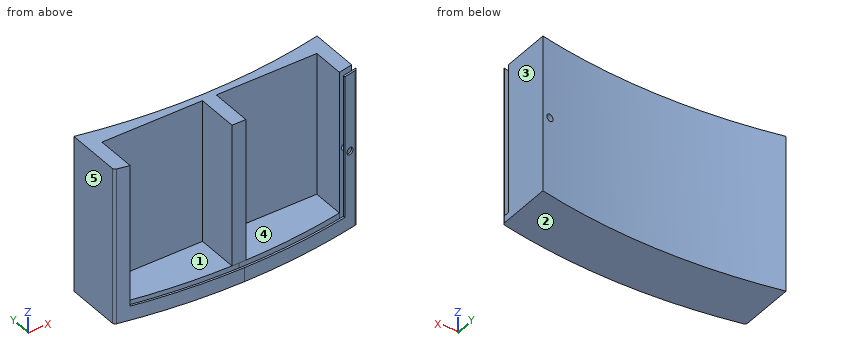
```python
from build123d import *

# Parameters (mm, degrees)
BOSS_EXTRUDE2_DEPTH     = 279.4
CUT_EXTRUDE1_DEPTH      = 279.4
FILLET1_R               = 2.54
SKETCH7_W               = 192.0875
SKETCH7_H               = 254
CUT_EXTRUDE2_DEPTH      = 44.45
SKETCH8_W               = 6.173248721
SKETCH8_H               = 35.639061591
BOSS_EXTRUDE3_DEPTH     = 258.064
CUT_EXTRUDE3_DEPTH      = 260.35
CUT_EXTRUDE3_DEPTH_BACK = 6.35
CUT_EXTRUDE4_DEPTH      = 260.35
CUT_EXTRUDE4_DEPTH_BACK = 6.35
BOSS_EXTRUDE4_DEPTH     = 254
SKETCH18_R              = 3.175
CUT_EXTRUDE5_DEPTH      = 71.12


with BuildPart() as part:
    # CrossSection → Boss-Extrude2 (new body)
    with BuildSketch(Plane.XY):
        with BuildLine():
            Line((108.74375, 11.322324676), (108.74375, -50.8))
            Line((108.74375, -50.8), (-108.74375, -50.8))
            Line((-108.74375, -50.8), (-108.74375, 11.322324676))
            ThreePointArc((-108.74375, 11.322324676), (0, 0), (108.74375, 11.322324676))
        make_face()
    extrude(amount=BOSS_EXTRUDE2_DEPTH)

    # Sketch4 → Cut-Extrude1 (cut)
    with BuildSketch(Plane(origin=(0, 0, 0), x_dir=(-1, 0, 0), z_dir=(0, 0, -1))):
        with BuildLine():
            ThreePointArc((0, -50.8), (-54.665798723, -47.96178867), (-108.74375, -39.477675324))
            Line((-108.74375, -39.477675324), (-108.74375, -50.8))
            Line((-108.74375, -50.8), (0, -50.8))
        make_face()
        with BuildLine():
            ThreePointArc((108.74375, -39.477675324), (54.665798723, -47.96178867), (0, -50.8))
            Line((0, -50.8), (108.74375, -50.8))
            Line((108.74375, -50.8), (108.74375, -39.477675324))
        make_face()
    extrude(amount=-CUT_EXTRUDE1_DEPTH, mode=Mode.SUBTRACT)

    # Fillet1
    fillet1_edges = [part.edges().sort_by_distance(p)[0] for p in [
        (108.74375, -39.477675324, 139.7),
        (-108.74375, -39.477675324, 139.7),
    ]]
    fillet(fillet1_edges, radius=FILLET1_R)

    # Sketch7 → Cut-Extrude2 (cut)
    with BuildSketch(Plane(origin=(0, -50.8, 0), x_dir=(1, 0, 0), z_dir=(0, 1, 0))):
        with Locations((0, -139.7)):
            Rectangle(SKETCH7_W, SKETCH7_H)
    extrude(amount=CUT_EXTRUDE2_DEPTH, mode=Mode.SUBTRACT)

    # Sketch8 → Boss-Extrude3 (add)
    with BuildSketch(Plane.XY.offset(12.7)):
        with Locations((3.086624361, -24.169530796)):
            Rectangle(SKETCH8_W, SKETCH8_H)
        with Locations((-3.086624361, -24.169530796)):
            Rectangle(SKETCH8_W, SKETCH8_H)
    extrude(amount=BOSS_EXTRUDE3_DEPTH)

    # Sketch13 → Cut-Extrude3 (cut, two sides: drawn at the far end of the back side and taken through both)
    with BuildSketch(Plane.XY.offset(12.7).offset(-CUT_EXTRUDE3_DEPTH_BACK)):
        with BuildLine():
            ThreePointArc((-96.04375, -40.123592373), (-48.223527841, -46.727181022), (0, -48.934530782))
            Line((0, -48.934530782), (0, -43.854530782))
            ThreePointArc((0, -43.854530782), (-48.223527841, -41.647181022), (-96.04375, -35.043592373))
            Line((-96.04375, -35.043592373), (-96.04375, -37.583592373))
            Line((-96.04375, -37.583592373), (-96.04375, -40.123592373))
        make_face()
        with BuildLine():
            Line((0, -43.854530782), (0, -48.934530782))
            ThreePointArc((0, -48.934530782), (48.223527841, -46.727181022), (96.04375, -40.123592373))
            Line((96.04375, -40.123592373), (96.04375, -37.583592373))
            Line((96.04375, -37.583592373), (96.04375, -35.043592373))
            ThreePointArc((96.04375, -35.043592373), (48.223527841, -41.647181022), (0, -43.854530782))
        make_face()
    extrude(amount=CUT_EXTRUDE3_DEPTH + CUT_EXTRUDE3_DEPTH_BACK, mode=Mode.SUBTRACT)

    # Sketch14 → Cut-Extrude4 (cut, two sides: drawn at the far end of the back side and taken through both)
    with BuildSketch(Plane(origin=(0, 0, 266.7), x_dir=(-1, 0, 0), z_dir=(0, 0, -1)).offset(-CUT_EXTRUDE4_DEPTH_BACK)):
        with BuildLine():
            Line((96.04375, -35.043592373), (96.04375, -40.123592373))
            ThreePointArc((96.04375, -40.123592373), (-28.026510339, -48.189989717), (-150.541934286, -27.012946445))
            Line((-150.541934286, -27.012946445), (-150.541934286, -21.932946445))
            ThreePointArc((-150.541934286, -21.932946445), (-28.026510339, -43.109989717), (96.04375, -35.043592373))
        make_face()
    extrude(amount=CUT_EXTRUDE4_DEPTH + CUT_EXTRUDE4_DEPTH_BACK, mode=Mode.SUBTRACT)

    # Sketch15 → Boss-Extrude4 (add)
    with BuildSketch(Plane(origin=(0, 0, 266.7), x_dir=(-1, 0, 0), z_dir=(0, 0, -1))):
        with BuildLine():
            Line((6.173248721, -43.818432493), (6.173248721, -41.989061591))
            Line((6.173248721, -41.989061591), (-6.173248721, -41.989061591))
            Line((-6.173248721, -41.989061591), (-6.173248721, -43.818432493))
            ThreePointArc((-6.173248721, -43.818432493), (0, -43.854530782), (6.173248721, -43.818432493))
        make_face()
    extrude(amount=BOSS_EXTRUDE4_DEPTH)

    # Sketch18 → Cut-Extrude5 (cut)
    with BuildSketch(Plane(origin=(0, -50.8, 0), x_dir=(1, 0, 0), z_dir=(0, 1, 0))):
        with Locations(Location((101.380501252, -209.55, 0), (0, 0, 90))):
            Circle(SKETCH18_R)
        with Locations(Location((101.380501252, -69.85, 0), (0, 0, 90))):
            Circle(SKETCH18_R)
    extrude(amount=CUT_EXTRUDE5_DEPTH, mode=Mode.SUBTRACT)


with BuildPart() as body_2:
    # Split2: the piece on the far side of the plane
    add(part.part)
    split(bisect_by=Plane.XY.offset(139.7), keep=Keep.BOTTOM)


with BuildPart() as part_1:
    add(part.part)

    # Split2
    split(bisect_by=Plane.XY.offset(139.7), keep=Keep.TOP)


solid = body_2.part
```
Verification items for the finished model (mm, model axes). Face numbers are marked on the shaded views. A direction names the side the tool comes from. Give positions to 0.01 mm unless a question says otherwise; leave off trailing zeros. Order: outer loops, then holes, each group sorted by start corner. A loop starts at its lowest first (then second) coordinate and runs counter-clockwise, first axis right, second up. Notation, with made-up numbers: (59.25, 3) -> (110.25, 3) arc R32 cw to (110.25, 41) -> close; hole circle Ø2 at (38.25, 25). An arc over 180 degrees is marked (long way). Use a Markdown table: item, result.
1) Depth check by flat-ended pin: pin 1 Ø6 at (x, y) = (48.5, -25.5) entering from +Z; pin 2 Ø1.5 at (x, y) = (64.5, -25.5) entering from -Z; pin 3 Ø4 at (x, z) = (-34.5, 29.5) entering from -Y; pin 4 Ø3 at (x, z) = (-83.5, 86.5) entering from +Y. Enter the tip coordinate at first touch or a pass-through.
Results:
| item | result |
|---|---|
| pin 1 | z = 12.7 |
| pin 2 | z = 0 |
| pin 3 | y = -6.35 |
| pin 4 | y = 6.89 |
2) Material ranges on probe 1 along X at (y, z) = (-21.5, 69.85); probe 2 along X at (y, z) = (-16.5, 75.5); probe 3 along X at (y, z) = (-39, 69), recorded low to high.
Results:
| item | result |
|---|---|
| probe 1 | -108.74 to -96.04, -6.17 to 6.17, 96.04 to 98.21, 104.56 to 108.74 |
| probe 2 | -108.74 to -96.04, -6.17 to 6.17, 96.04 to 108.74 |
| probe 3 | -108.19 to -96.04, -6.17 to 6.17, 104.44 to 108.19 |
3) Mould release check, pull along X, two halves, no side actions. Record for the marked faces 1, 2 and 3: pulls with the +X half, pulls with the -X half, needs draft (parallel to the pull), parting line crosses it, or undercut.
Results:
| item | result |
|---|---|
| face 1 | undercut |
| face 2 | needs draft |
| face 3 | pulls with the +X half |
4) Section check C-C, the plane z = 9. Record the boundary of the cut face in (x, y), then the cut area to 3 significant figures.
Results:
| item | result |
|---|---|
| outline | (-108.74, -37.41) arc R2.54 ccw to (-106.72, -39.9) arc R527.87 ccw to (106.72, -39.9) arc R2.54 ccw to (108.74, -37.61) arc R527.87 cw to (-96.04, -40.12) -> (-96.04, -35.04) arc R527.87 ccw to (108.74, -32.53) -> (108.74, 11.32) arc R527.87 cw to (-108.74, 11.32) -> close |
| area | 10,000 mm² |
5) Tool access check on the marked faces 4 and 5. Record the directions out of +Z, -Z, +X, -X, +Y, -Y that give a thin tool (end or side, any length) a straight path to the whole face; none if there is none.
Results:
| item | result |
|---|---|
| face 4 | +Z, -Y |
| face 5 | +Z, -Z, -X, +Y, -Y |
6) Section check B-B, the plane z = 61. Record the boundary of the cut face in (x, y).
Results:
| item | result |
|---|---|
| outline | (-108.74, -37.41) arc R2.54 ccw to (-106.72, -39.9) arc R527.87 ccw to (-96.04, -41.99) -> (-96.04, -6.35) -> (-6.17, -6.35) -> (-6.17, -43.82) arc R527.87 ccw to (6.17, -43.82) -> (6.17, -6.35) -> (96.04, -6.35) -> (96.04, -35.04) arc R527.87 ccw to (108.74, -32.53) -> (108.74, 11.32) arc R527.87 cw to (-108.74, 11.32) -> close; (96.04, -41.99) arc R527.87 ccw to (106.72, -39.9) arc R2.54 ccw to (108.74, -37.61) arc R527.87 cw to (96.04, -40.12) -> close |
